```python
from build123d import *

# Parameters (mm, degrees)
F0_W     = 400
F0_H     = 400
F1_DEPTH = 10
F2_R     = 12.898904
F3_DEPTH = 13


with BuildPart() as f1:
    # F0 (on Top) → F1 (new body)
    with BuildSketch(Plane.XY):
        Rectangle(F0_W, F0_H)
    extrude(amount=F1_DEPTH)

    # F2 (on face) → F3 (cut)
    with BuildSketch(Plane.XY.offset(10)):
        with Locations((164.230794, -176.38047)):
            Circle(F2_R)
        with Locations((164.230794, -137.38047)):
            Circle(F2_R)
        with Locations((164.230794, -98.38047)):
            Circle(F2_R)
        with Locations((164.230794, -59.38047)):
            Circle(F2_R)
        with Locations((164.230794, -20.38047)):
            Circle(F2_R)
        with Locations((164.230794, 18.61953)):
            Circle(F2_R)
        with Locations((164.230794, 57.61953)):
            Circle(F2_R)
        with Locations((164.230794, 96.61953)):
            Circle(F2_R)
        with Locations((164.230794, 135.61953)):
            Circle(F2_R)
        with Locations((164.230794, 174.61953)):
            Circle(F2_R)
        with Locations((126.230794, -176.38047)):
            Circle(F2_R)
        with Locations((126.230794, -137.38047)):
            Circle(F2_R)
        with Locations((126.230794, -98.38047)):
            Circle(F2_R)
        with Locations((126.230794, -59.38047)):
            Circle(F2_R)
        with Locations((126.230794, -20.38047)):
            Circle(F2_R)
        with Locations((126.230794, 18.61953)):
            Circle(F2_R)
        with Locations((126.230794, 57.61953)):
            Circle(F2_R)
        with Locations((126.230794, 96.61953)):
            Circle(F2_R)
        with Locations((126.230794, 135.61953)):
            Circle(F2_R)
        with Locations((126.230794, 174.61953)):
            Circle(F2_R)
        with Locations((88.230794, -176.38047)):
            Circle(F2_R)
        with Locations((88.230794, -137.38047)):
            Circle(F2_R)
        with Locations((88.230794, -98.38047)):
            Circle(F2_R)
        with Locations((88.230794, -59.38047)):
            Circle(F2_R)
        with Locations((88.230794, -20.38047)):
            Circle(F2_R)
        with Locations((88.230794, 18.61953)):
            Circle(F2_R)
        with Locations((88.230794, 57.61953)):
            Circle(F2_R)
        with Locations((88.230794, 96.61953)):
            Circle(F2_R)
        with Locations((88.230794, 135.61953)):
            Circle(F2_R)
        with Locations((88.230794, 174.61953)):
            Circle(F2_R)
        with Locations((50.230794, -176.38047)):
            Circle(F2_R)
        with Locations((50.230794, -137.38047)):
            Circle(F2_R)
        with Locations((50.230794, -98.38047)):
            Circle(F2_R)
        with Locations((50.230794, -59.38047)):
            Circle(F2_R)
        with Locations((50.230794, -20.38047)):
            Circle(F2_R)
        with Locations((50.230794, 18.61953)):
            Circle(F2_R)
        with Locations((50.230794, 57.61953)):
            Circle(F2_R)
        with Locations((50.230794, 96.61953)):
            Circle(F2_R)
        with Locations((50.230794, 135.61953)):
            Circle(F2_R)
        with Locations((50.230794, 174.61953)):
            Circle(F2_R)
        with Locations((12.230794, -176.38047)):
            Circle(F2_R)
        with Locations((12.230794, -137.38047)):
            Circle(F2_R)
        with Locations((12.230794, -98.38047)):
            Circle(F2_R)
        with Locations((12.230794, -59.38047)):
            Circle(F2_R)
        with Locations((12.230794, -20.38047)):
            Circle(F2_R)
        with Locations((12.230794, 18.61953)):
            Circle(F2_R)
        with Locations((12.230794, 57.61953)):
            Circle(F2_R)
        with Locations((12.230794, 96.61953)):
            Circle(F2_R)
        with Locations((12.230794, 135.61953)):
            Circle(F2_R)
        with Locations((12.230794, 174.61953)):
            Circle(F2_R)
        with Locations((-25.769206, -176.38047)):
            Circle(F2_R)
        with Locations((-25.769206, -137.38047)):
            Circle(F2_R)
        with Locations((-25.769206, -98.38047)):
            Circle(F2_R)
        with Locations((-25.769206, -59.38047)):
            Circle(F2_R)
        with Locations((-25.769206, -20.38047)):
            Circle(F2_R)
        with Locations((-25.769206, 18.61953)):
            Circle(F2_R)
        with Locations((-25.769206, 57.61953)):
            Circle(F2_R)
        with Locations((-25.769206, 96.61953)):
            Circle(F2_R)
        with Locations((-25.769206, 135.61953)):
            Circle(F2_R)
        with Locations((-25.769206, 174.61953)):
            Circle(F2_R)
        with Locations((-63.769206, -176.38047)):
            Circle(F2_R)
        with Locations((-63.769206, -137.38047)):
            Circle(F2_R)
        with Locations((-63.769206, -98.38047)):
            Circle(F2_R)
        with Locations((-63.769206, -59.38047)):
            Circle(F2_R)
        with Locations((-63.769206, -20.38047)):
            Circle(F2_R)
        with Locations((-63.769206, 18.61953)):
            Circle(F2_R)
        with Locations((-63.769206, 57.61953)):
            Circle(F2_R)
        with Locations((-63.769206, 96.61953)):
            Circle(F2_R)
        with Locations((-63.769206, 135.61953)):
            Circle(F2_R)
        with Locations((-63.769206, 174.61953)):
            Circle(F2_R)
        with Locations((-101.769206, -176.38047)):
            Circle(F2_R)
        with Locations((-101.769206, -137.38047)):
            Circle(F2_R)
        with Locations((-101.769206, -98.38047)):
            Circle(F2_R)
        with Locations((-101.769206, -59.38047)):
            Circle(F2_R)
        with Locations((-101.769206, -20.38047)):
            Circle(F2_R)
        with Locations((-101.769206, 18.61953)):
            Circle(F2_R)
        with Locations((-101.769206, 57.61953)):
            Circle(F2_R)
        with Locations((-101.769206, 96.61953)):
            Circle(F2_R)
        with Locations((-101.769206, 135.61953)):
            Circle(F2_R)
        with Locations((-101.769206, 174.61953)):
            Circle(F2_R)
        with Locations((-139.769206, -176.38047)):
            Circle(F2_R)
        with Locations((-139.769206, -137.38047)):
            Circle(F2_R)
        with Locations((-139.769206, -98.38047)):
            Circle(F2_R)
        with Locations((-139.769206, -59.38047)):
            Circle(F2_R)
        with Locations((-139.769206, -20.38047)):
            Circle(F2_R)
        with Locations((-139.769206, 18.61953)):
            Circle(F2_R)
        with Locations((-139.769206, 57.61953)):
            Circle(F2_R)
        with Locations((-139.769206, 96.61953)):
            Circle(F2_R)
        with Locations((-139.769206, 135.61953)):
            Circle(F2_R)
        with Locations((-139.769206, 174.61953)):
            Circle(F2_R)
        with Locations((-177.769206, -176.38047)):
            Circle(F2_R)
        with Locations((-177.769206, -137.38047)):
            Circle(F2_R)
        with Locations((-177.769206, -98.38047)):
            Circle(F2_R)
        with Locations((-177.769206, -59.38047)):
            Circle(F2_R)
        with Locations((-177.769206, -20.38047)):
            Circle(F2_R)
        with Locations((-177.769206, 18.61953)):
            Circle(F2_R)
        with Locations((-177.769206, 57.61953)):
            Circle(F2_R)
        with Locations((-177.769206, 96.61953)):
            Circle(F2_R)
        with Locations((-177.769206, 135.61953)):
            Circle(F2_R)
        with Locations((-177.769206, 174.61953)):
            Circle(F2_R)
    extrude(amount=-F3_DEPTH, mode=Mode.SUBTRACT)


solid = f1.part
```
Verification items for the finished model (mm, model axes). Round coordinates to 2 decimals unless told otherwise and drop trailing zeros. Answer as a JSON object with one key per item and string values. Group by question number.
Q1. Section check A-A, the plane x = 161.5. Give the number of separate pieces and of enclosed holes in the cut face, plus the area to 3 significant figures.
Q2. Mould release check, pull along X, two halves, no side actions. Record for faces 1 (the cylindrical face through (116.724, 183.337, 5.07)), 2 (the flat face through (-3, -200, 5)): released by +X, released by -X, zero draft, split by the parting line, or undercut.
Q3. Go/stop test with a flat-tipped pin: pin 1 Ø1.5 at (x, y) = (99, -62.5) entering from +Z. Record where the tip stops, or that it passes through.
Found:
{
 "1": {"separate pieces": "11", "enclosed holes": "0", "area": "1,480 mm^2"},
 "2": {"face 1": "undercut", "face 2": "zero draft"},
 "3": {"pin 1": "passes through"}
}
